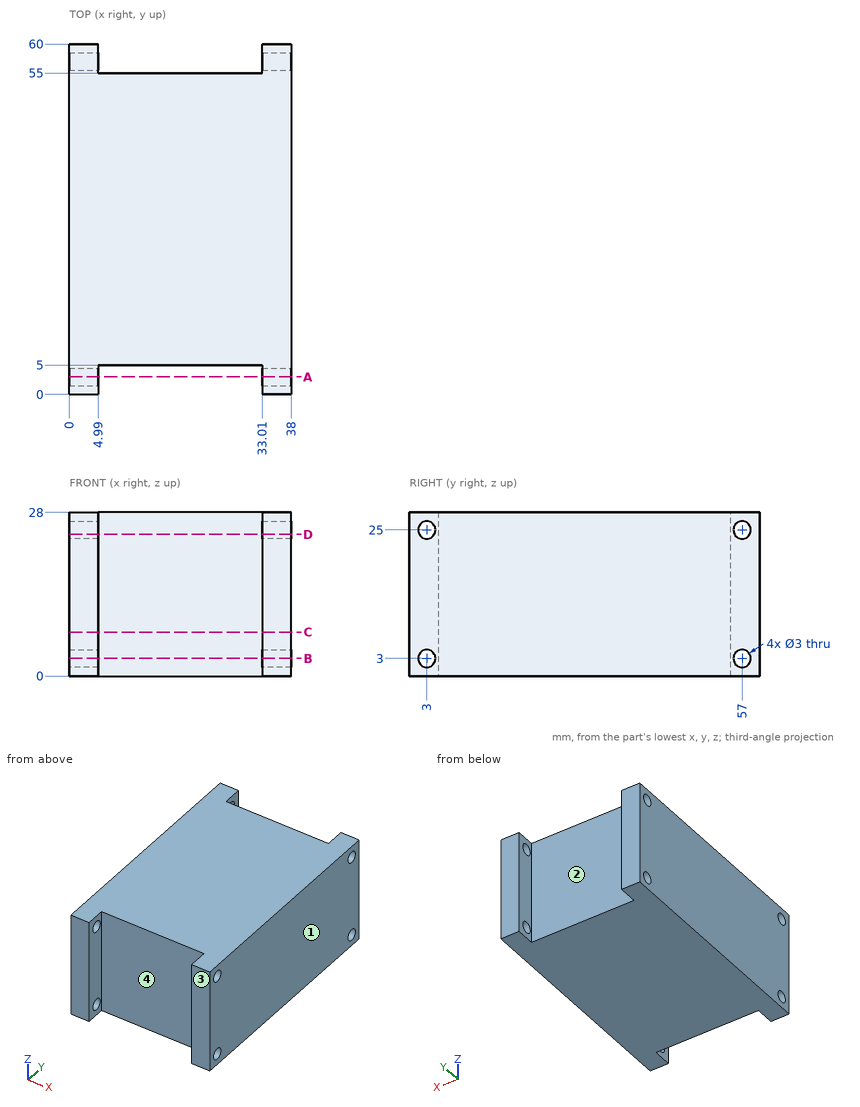
Study the drawing (mm; zero at the part's minimum x, y, z) and answer. Give positions to 0.01 mm unless a question says otherwise; leave off trailing zeros. Order: outer loops, then holes, each group sorted by start corner. A loop starts at its lowest first (then second) coordinate and runs counter-clockwise, first axis right, second up. Notation, with made-up numbers: (24.5, 77) - (75.5, 77) arc R9 ccw to (75.5, 91) - close; hole circle Ø11 at (-4.5, 44.5). An arc over 180 degrees is marked (long way). Use one line per item in the form item = value. Start each with the question number.
(1) A cutting plane is placed at D-D, the plane z = 24.25. Write down the section's boundary in (x, y), then the cut area to 3 significant figures.
(2) A cutting plane is placed at B-B, the plane z = 3. Write down the section's boundary in (x, y).
(3) A cutting plane is placed at C-C, the plane z = 7.5. Write down the section's boundary in (x, y).
(4) Flat-ended cylindrical pins translate along their axes: pin 1 Ø2 at (x, z) = (9.5, 10.5) entering from +Y; pin 2 Ø1 at (x, z) = (14.5, 17) entering from -Y; pin 3 Ø5.5 at (y, z) = (2, 12.5) entering from -X. Find the tip coordinate at first contact, or state that the pin passes through.
(5) The mould has two halves that part along X. Classify the marked faces 1, 2, 3 and 4: released by +X, released by -X, zero draft, split by the parting line, or undercut.
(6) Consider line 1 (Y direction, x = 3.3, z = 25); line 2 (Z direction, x = 3.5, y = 3.5); line 3 (X direction, y = 57, z = 16.5). Determine where each line is inside the solid, lowest interval first. Write a range as from..to.
(7) A cutting plane is placed at A-A, the plane y = 3. Write down the section's boundary in (x, z).
Ans:
q1.outline = (0, 0) - (4.99, 0) - (4.99, 1.7) - (0, 1.7) - close; (0, 4.3) - (4.99, 4.3) - (4.99, 5) - (33.01, 5) - (33.01, 4.3) - (38, 4.3) - (38, 55.7) - (33.01, 55.7) - (33.01, 55) - (4.99, 55) - (4.99, 55.7) - (0, 55.7) - close; (0, 58.3) - (4.99, 58.3) - (4.99, 60) - (0, 60) - close; (33.01, 0) - (38, 0) - (38, 1.7) - (33.01, 1.7) - close; (33.01, 58.3) - (38, 58.3) - (38, 60) - (33.01, 60) - close
q1.area = 1,950 mm^2
q2.outline = (0, 0) - (4.99, 0) - (4.99, 1.5) - (0, 1.5) - close; (0, 4.5) - (4.99, 4.5) - (4.99, 5) - (33.01, 5) - (33.01, 4.5) - (38, 4.5) - (38, 55.5) - (33.01, 55.5) - (33.01, 55) - (4.99, 55) - (4.99, 55.5) - (0, 55.5) - close; (0, 58.5) - (4.99, 58.5) - (4.99, 60) - (0, 60) - close; (33.01, 0) - (38, 0) - (38, 1.5) - (33.01, 1.5) - close; (33.01, 58.5) - (38, 58.5) - (38, 60) - (33.01, 60) - close
q3.outline = (0, 0) - (4.99, 0) - (4.99, 5) - (33.01, 5) - (33.01, 0) - (38, 0) - (38, 60) - (33.01, 60) - (33.01, 55) - (4.99, 55) - (4.99, 60) - (0, 60) - close
q4.pin_1 = 55
q4.pin_2 = 5
q4.pin_3 = 0
q5.face_1 = released by +X
q5.face_2 = undercut
q5.face_3 = zero draft
q5.face_4 = undercut
q6.line_1 = 0..1.5, 4.5..55.5, 58.5..60
q6.line_2 = 0..1.59, 4.41..23.59, 26.41..28
q6.line_3 = 0..4.99, 33.01..38
q7.outline = (0, 0) - (4.99, 0) - (4.99, 1.5) - (0, 1.5) - close; (0, 4.5) - (4.99, 4.5) - (4.99, 23.5) - (0, 23.5) - close; (0, 26.5) - (4.99, 26.5) - (4.99, 28) - (0, 28) - close; (33.01, 0) - (38, 0) - (38, 1.5) - (33.01, 1.5) - close; (33.01, 4.5) - (38, 4.5) - (38, 23.5) - (33.01, 23.5) - close; (33.01, 26.5) - (38, 26.5) - (38, 28) - (33.01, 28) - close
